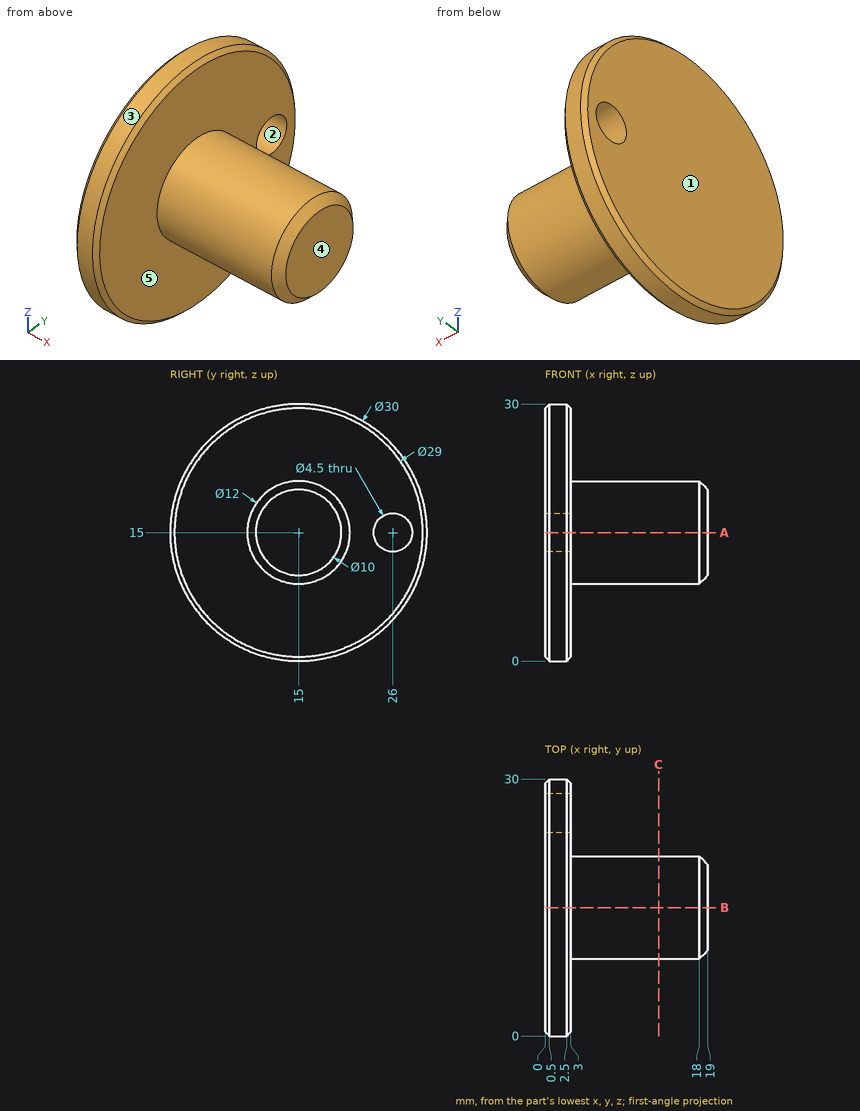
The figure shows three views and two pictorial views of one solid part (mm, origin at its lowest corner). Answer the questions. A direction names the side the tool comes from. Coordinates: 2 decimals unless noted, no trailing zeros. Loops run counter-clockwise (first coordinate to the right, second up) from the corner with the lowest first, then second, coordinate; pieces in that order, holes last.
1) Flat-ended cylindrical pins translate along their axes: pin 1 Ø1 at (x, y) = (15, 22.5) entering from +Z; pin 2 Ø2 at (x, z) = (6, 18.5) entering from +Y; pin 3 Ø5 at (x, z) = (16, 10) entering from -Y; pin 4 Ø8 at (x, y) = (5, 21) entering from +Z. Find the tip coordinate at first contact, or state that the pin passes through.
2) A tool of negligible diameter and unlimited length cuts with its end or side. For the marked faces 4 and 5, from which of +Z, -Z, +X, -X, +Y, -Y can it reach the whole face along a straight path? Write none if from no direction.
3) Determine the mould class of the marked faces 1, 2 and 3 for opening direction Y: pulls with the +Y half, pulls with the -Y half, needs draft (parallel to the pull), parting line crosses it, or undercut.
4) Find section A-A on z = 15. Write down the section's boundary in (x, y).
5) Find section C-C on x = 13.25. Write down the section's boundary in (y, z).
6) Find the intervals of material crossed by L1, parallel to Y at x = 1.65, z = 15; L2, parallel to X at y = 2, z = 16; L3, parallel to Z at x = 11.75, y = 19.25, in increasing order.
7) Find section B-B on y = 15. Write down the section's boundary in (x, z).
Values:
1. pin 1: passes through
1. pin 2: stops at y = 20.45
1. pin 3: stops at y = 9.55
1. pin 4: stops at z = 29.72
2. face 4: +Z, -Z, +X, +Y, -Y
2. face 5: +X
3. face 1: needs draft
3. face 2: undercut
3. face 3: parting line crosses it
4. outline: (0, 0.5) - (0.5, 0) - (2.5, 0) - (3, 0.5) - (3, 9) - (18, 9) - (19, 10) - (19, 20) - (18, 21) - (3, 21) - (3, 23.75) - (0, 23.75) - close; (0, 28.25) - (3, 28.25) - (3, 29.5) - (2.5, 30) - (0.5, 30) - (0, 29.5) - close
5. outline: circle Ø12 at (15, 15)
6. L1: y = 0 to 23.75, 28.25 to 30
6. L2: x = 0 to 3
6. L3: z = 10.76 to 19.24
7. outline: (0, 0.5) - (0.5, 0) - (2.5, 0) - (3, 0.5) - (3, 9) - (18, 9) - (19, 10) - (19, 20) - (18, 21) - (3, 21) - (3, 29.5) - (2.5, 30) - (0.5, 30) - (0, 29.5) - close
